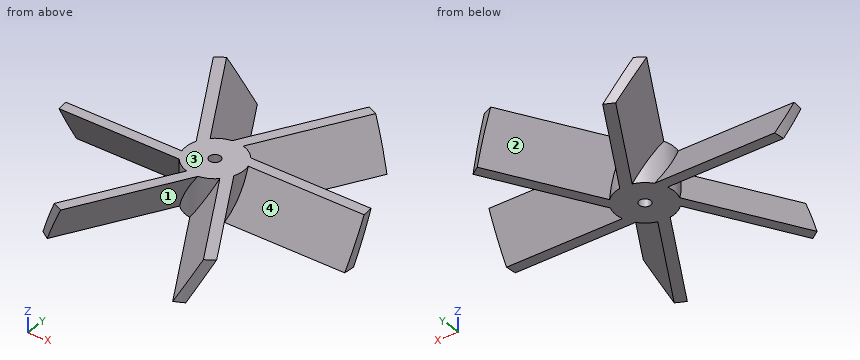
```python
from build123d import *

# Parameters (mm, degrees)
F0_R            = 6.35
F0_R_2          = 1.24968
F1_DEPTH        = 4.7625
F4_COPIES_COUNT = 6
F5_R            = 254
F5_R_2          = 31.75
F6_DEPTH        = 9.526


# Not quite as in the source:
# - a pattern or mirror of a feature is missing from the dataset's text; its kind, count and spacing are read off the source's solid


with BuildPart() as f1:
    # F0 (on Top) → F1 (new body, symmetric)
    with BuildSketch(Plane.XY):
        Circle(F0_R)
        Circle(F0_R_2, mode=Mode.SUBTRACT)
    extrude(amount=F1_DEPTH, both=True)

    # F3 (on offset) → F4 (join, up to the next surface of F1)
    with BuildSketch(Plane.YZ.offset(152.4)):
        Polygon((1.57645491, 4.7625), (-3.922806404, -4.7625), (-1.57645491, -4.7625), (3.922806404, 4.7625), align=None)
    f4 = extrude(until=Until.NEXT, dir=(-1, 0, 0))

    # F4_copies: F4 ×6 about axis
    f4_copies_axis = Axis((0, 0, 0), (0, 0, 1))
    for i in range(1, F4_COPIES_COUNT):
        add(f4.rotate(f4_copies_axis, i * 360 / F4_COPIES_COUNT))

    # F5 (on face) → F6 (cut, through all)
    with BuildSketch(Plane.XY.offset(4.7625)):
        Circle(F5_R)
        Circle(F5_R_2, mode=Mode.SUBTRACT)
    extrude(amount=-F6_DEPTH, mode=Mode.SUBTRACT)


solid = f1.part
```
Input: part model. Units: mm. Frame: model coordinates. Face numbers are marked on the shaded views. Round coordinates to 2 decimals unless told otherwise and drop trailing zeros. Order: outer loops, then holes, each group sorted by start corner. A loop starts at its lowest first (then second) coordinate and runs counter-clockwise, first axis right, second up. Notation, with made-up numbers: (-37.5, 64.25) - (-2.5, 64.25) arc R21 cw to (-2.5, 68.25) - close; hole circle Ø11 at (37, -12). An arc over 180 degrees is marked (long way). One line per question, with ' | ' between items. Start each with the question number.
1) Cut plane A-A, the plane y = -21. Return the cut outline in (x, z), then the cut area to 3 significant figures.
2) Ray query, probe 1 along Y at (x, z) = (0, 1.25); probe 2 along X at (y, z) = (-25, 0.25); probe 3 along Y at (x, z) = (14, -0.5) (1 decimal). Return the intervals inside material, ascending.
3) Contact query for flat-ended pins moving along their axis: P1, Ø2, axis at y = -6.5, z = -1, coming from the -X side; P2, Ø4, axis at x = 0, y = 0, coming from the -Z side; P3, Ø5, axis at y = -18.5, z = 1.5, coming from the +X side; P4, Ø1, axis at y = 2, z = -0.5, coming from the +X side. Output: stop coordinate, or through.
4) Cut plane D-D, the plane x = 0. Return the cut outline in (y, z).
5) Pull-direction query (Y, two-part tool) for the marked faces 1, 2, 3 and 4; classes: +Y half, -Y half, draft (parallel to the pull), parting line (faces both ways), or undercut.
6) Cut plane C-C, the plane x = -9. Return the cut outline in (y, z), then the cut area to 3 significant figures.
7) Cut plane B-B, the plane z = -1.25. Return the cut outline in (x, y), then the cut area to 3 significant figures.
Worked out:
1) outline: (-16.65, -4.76) - (-13.94, -4.76) - (-7.59, 4.76) - (-10.3, 4.76) - close; (7.59, -4.76) - (10.3, -4.76) - (16.65, 4.76) - (13.94, 4.76) - close | area: 51.6 mm^2
2) probe 1: y = -6.35 to -1.25, 1.25 to 6.35 | probe 2: x = -15.62 to -12.91, 13.25 to 15.96 | probe 3: y = -27.2 to -22.5, -1.5 to 0.9, 21.3 to 26
3) P1: stops at x = -6.66 | P2: stops at z = -4.76 | P3: stops at x = 15.24 | P4: stops at x = 6.17
4) outline: (-7.85, -4.76) - (-1.25, -4.76) - (-1.25, 4.76) - (-7.85, 4.76) - (-6.35, 3.47) - (-6.35, -3.47) - close; (1.25, -4.76) - (7.85, -4.76) - (6.35, -3.47) - (6.35, 3.47) - (7.85, 4.76) - (1.25, 4.76) - close
5) face 1: -Y half | face 2: +Y half | face 3: draft | face 4: undercut
6) outline: (-23.43, 4.76) - (-12.44, -4.76) - (-7.74, -4.76) - (-18.74, 4.76) - close; (-3.92, 4.76) - (1.58, -4.76) - (3.92, -4.76) - (-1.58, 4.76) - close; (7.74, 4.76) - (18.74, -4.76) - (23.43, -4.76) - (12.44, 4.76) - close | area: 112 mm^2
7) outline: (-31.75, -0.45) - (-6.33, -0.45) arc R6.35 ccw to (-4.67, -4.3) - (-17.49, -26.5) arc R31.75 ccw to (-15.48, -27.72) - (-2.78, -5.71) arc R6.35 ccw to (1.39, -6.2) - (14.21, -28.39) arc R31.75 ccw to (16.26, -27.27) - (3.56, -5.26) arc R6.35 ccw to (6.06, -1.89) - (31.69, -1.89) arc R31.75 ccw to (31.75, 0.45) - (6.33, 0.45) arc R6.35 ccw to (4.67, 4.3) - (17.49, 26.5) arc R31.75 ccw to (15.48, 27.72) - (2.78, 5.71) arc R6.35 ccw to (-1.39, 6.2) - (-14.21, 28.39) arc R31.75 ccw to (-16.26, 27.27) - (-3.56, 5.26) arc R6.35 ccw to (-6.06, 1.89) - (-31.69, 1.89) arc R31.75 ccw to start; hole circle Ø2.5 at (0, 0) | area: 480 mm^2
